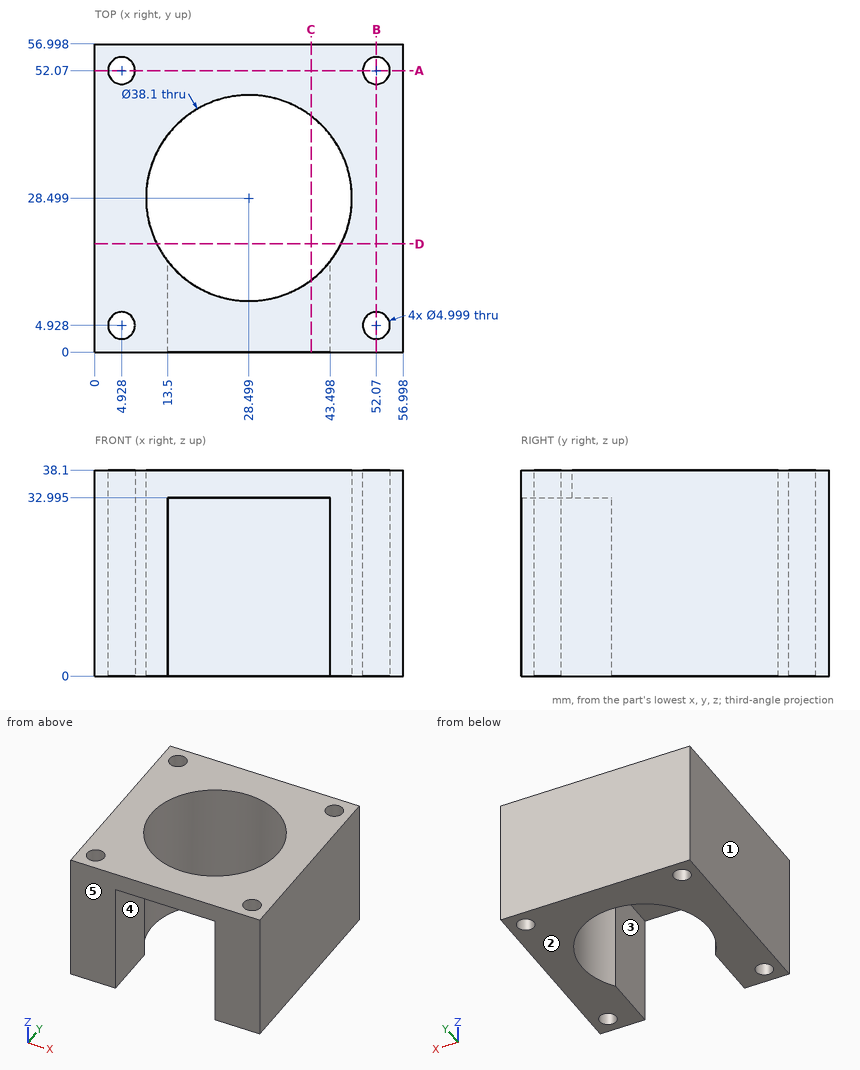
Source: three-view drawing plus pictorial views. Frame: mm from the lowest corner of the part. A direction names the side the tool comes from. Coordinates: 2 decimals unless noted, no trailing zeros. Write each loop counter-clockwise with the first axis right and the second up, starting at its lowest first coordinate (ties: lowest second). Pieces come first, ordered by that corner, then holes. Notation, with made-up numbers: (46, -23.5) - (102, -23.5) arc R8 cw to (102, -11.5) - close; hole circle Ø7 at (70, 15). An arc over 180 degrees is marked (long way). Return JSON: item names as keys, results as strings.
Item 1: Section query A-A (y = 52.07). Output: boundary loops of the cut face in (x, z), and give its area (3 significant figures).
Completed:
{"outline": "(0, 0) - (2.43, 0) - (2.43, 38.1) - (0, 38.1) - close; (7.43, 0) - (49.57, 0) - (49.57, 38.1) - (7.43, 38.1) - close; (54.57, 0) - (57, 0) - (57, 38.1) - (54.57, 38.1) - close", "area": "1,790 mm2"}
Item 2: Section query D-D (y = 20). Output: boundary loops of the cut face in (x, z).
Completed:
{"outline": "(0, 0) - (11.45, 0) - (11.45, 38.1) - (0, 38.1) - close; (45.55, 0) - (57, 0) - (57, 38.1) - (45.55, 38.1) - close"}
Item 3: Reachability of the marked faces 4 and 5 from +Z, -Z, +X, -X, +Y, -Y: full face, straight path, thin tool, end or side. Return the list, or none.
Completed:
{"face 4": "-Z, -Y", "face 5": "+Z, -Z, +X, -X, -Y"}
Item 4: Section query C-C (x = 40). Output: boundary loops of the cut face in (y, z) (1 decimal).
Completed:
{"outline": "(0, 33) - (13.3, 33) - (13.3, 38.1) - (0, 38.1) - close; (43.7, 0) - (57, 0) - (57, 38.1) - (43.7, 38.1) - close"}
Item 5: Line query: L1, parallel to X at y = 5, z = 21 (1 decimal); L2, parallel to Y at x = 52.07, z = 8; L3, parallel to X at y = 10, z = 25.5. Output: solid intervals per line, ascending.
Completed:
{"L1": "x = 0 to 2.4, 7.4 to 13.5, 43.5 to 49.6, 54.6 to 57", "L2": "y = 0 to 2.43, 7.43 to 49.57, 54.57 to 57", "L3": "x = 0 to 13.5, 43.5 to 57"}
Item 6: Pull-direction query (X, two-part tool) for the marked faces 1, 2 and 3; classes: +X half, -X half, draft (parallel to the pull), parting line (faces both ways), or undercut.
Completed:
{"face 1": "-X half", "face 2": "draft", "face 3": "undercut"}
Item 7: Pin query (flat end, axial travel): pin 1 Ø8.5 at (y, z) = (11, 13.5) entering from -X; pin 2 Ø18.5 at (x, y) = (34, 11.5) entering from -Z (1 decimal). Return the tip coordinate at first contact, or that it passes through.
Completed:
{"pin 1": "stops at x = 0", "pin 2": "stops at z = 33"}
